Geometry check sheet. Reference: the model listing, model coordinates, mm. A direction names the side the tool comes from. Give positions to 0.01 mm unless a question says otherwise; leave off trailing zeros. Write each loop counter-clockwise with the first axis right and the second up, starting at its lowest first coordinate (ties: lowest second). Pieces come first, ordered by that corner, then holes.
(1) Cross-section at B-B (x = 8). Record the boundary of the cut face in (y, z), and give its area (3 significant figures).
(2) Tool access check on faces 5 (the flat face through (13, 27, -9)), 6 (the flat face through (30, -15, -2)). Record the directions out of +Z, -Z, +X, -X, +Y, -Y that give a thin tool (end or side, any length) a straight path to the whole face; none if there is none.
(3) Thickness scan on line 1 along Y through (x, z) = (8, -18.1); line 2 along X through (y, z) = (10, -38); line 3 along Y through (x, z) = (41, -2). Record the ranges inside material, lowest first.
(4) Depth check by flat-ended pin: P1, Ø3, axis at x = 33, z = -22.5, coming from the -Y side; P2, Ø2, axis at y = 10.5, z = -11, coming from the -X side; P3, Ø6, axis at y = 38.5, z = -32.5, coming from the +X side. Enter the tip coordinate at first touch or a pass-through.
(5) Cross-section at A-A (y = 10). Count the separate pieces of the cut face and the enclosed holes in it, and give its area (3 significant figures).
(6) Cross-section at C-C (y = 19). Record the boundary of the cut face in (x, z), and give its area (4 significant figures).
(7) Mould release check, pull along Y, two halves, no side actions. Record for faces 1 (the cylindrical face through (32.39, 24.43, -22.6)), 2 (the flat face through (12, 20, -20)), 3 (the flat face through (30, 55, -2)), 4 (the flat face through (33, 20, -22)): +Y half, -Y half, draft (parallel to the pull), parting line (faces both ways), or undercut.
(8) Cross-section at D-D (z = -43.5). Record the boundary of the cut face in (x, y).
```python
from build123d import *

# Parameters (mm, degrees)
SKETCH1_W                = 40
SKETCH1_H                = 40
BOSS_EXTRUDE1_DEPTH      = 40
SKETCH2_W                = 25
SKETCH2_H                = 20
CUT_EXTRUDE1_DEPTH       = 40
CHAMFER1_SIZE            = 15
CUT_EXTRUDE2_DEPTH       = 15
CHAMFER2_SIZE            = 4
SKETCH4_R                = 2.6
CUT_EXTRUDE3_DEPTH       = 17
BOSS_EXTRUDE2_DEPTH      = 8
BOSS_EXTRUDE2_DEPTH_BACK = 40
SKETCH5_W                = 40
SKETCH5_H                = 7
CHAMFER3_SIZE            = 35
CHAMFER3_SIZE2           = 25
CHAMFER4_SIZE            = 25
CHAMFER4_SIZE2           = 35
CHAMFER5_SIZE            = 8
FILLET1_R                = 10
FILLET2_R                = 5
SKETCH8_R                = 2.6
CUT_EXTRUDE4_DEPTH       = 34
BOSS_EXTRUDE3_DEPTH      = 20
FILLET3_R                = 4
FILLET4_R                = 2
CUT_EXTRUDE5_DEPTH       = 26
CHAMFER6_SIZE            = 2
CHAMFER6_SIZE2           = 10
FILLET5_R                = 2


with BuildPart() as part:
    # Sketch1 → Boss-Extrude1 (new body)
    with BuildSketch(Plane(origin=(0, 0, 0), x_dir=(1, 0, 0), z_dir=(0, 1, 0))):
        with Locations((20, 20)):
            Rectangle(SKETCH1_W, SKETCH1_H)
    extrude(amount=BOSS_EXTRUDE1_DEPTH)

    # Sketch2 → Cut-Extrude1 (cut)
    with BuildSketch(Plane(origin=(0, 40, 0), x_dir=(1, 0, 0), z_dir=(0, 1, 0))):
        with Locations((12.5, 30)):
            Rectangle(SKETCH2_W, SKETCH2_H)
    extrude(amount=-CUT_EXTRUDE1_DEPTH, mode=Mode.SUBTRACT)

    # Chamfer1
    chamfer1_edges = [part.edges().sort_by_distance(p)[0] for p in [
        (0, 20, 0),
    ]]
    chamfer(chamfer1_edges, length=CHAMFER1_SIZE)

    # Sketch3 → Cut-Extrude2 (cut)
    with BuildSketch(Plane.XY):
        Polygon((0, 10), (0, 15), (15, 15), (15, 5), (0, 5), align=None)
        Polygon((0, 30), (0, 25), (15, 25), (15, 35), (0, 35), align=None)
    extrude(amount=-CUT_EXTRUDE2_DEPTH, mode=Mode.SUBTRACT)

    # Chamfer2
    chamfer2_edges = [part.edges().sort_by_distance(p)[0] for p in [
        (15, 35, -7.5),
        (15, 25, -7.5),
        (15, 15, -7.5),
        (15, 5, -7.5),
    ]]
    chamfer(chamfer2_edges, length=CHAMFER2_SIZE)

    # Sketch4 → Cut-Extrude3 (cut)
    with BuildSketch(Plane.XY.offset(-15)):
        with Locations((8, 30)):
            Circle(SKETCH4_R)
        with Locations((8, 10)):
            Circle(SKETCH4_R)
    extrude(amount=-CUT_EXTRUDE3_DEPTH, mode=Mode.SUBTRACT)

    # Sketch5 → Boss-Extrude2 (add, two sides: drawn at the far end of the back side and taken through both)
    with BuildSketch(Plane(origin=(0, 0, -40), x_dir=(-1, 0, 0), z_dir=(0, 0, -1)).offset(-BOSS_EXTRUDE2_DEPTH_BACK)):
        with Locations((-60, 11.5)):
            Rectangle(SKETCH5_W, SKETCH5_H)
        with Locations((-60, 28.5)):
            Rectangle(SKETCH5_W, SKETCH5_H)
    extrude(amount=BOSS_EXTRUDE2_DEPTH + BOSS_EXTRUDE2_DEPTH_BACK)

    # Chamfer3
    chamfer3_edges = [part.edges().sort_by_distance(p)[0] for p in [
        (80, 28.5, 0),
    ]]
    chamfer3_side = [part.faces().sort_by_distance(p)[0] for p in [
        (39.166666667, 20, 0),
    ]]
    chamfer(chamfer3_edges, length=CHAMFER3_SIZE, length2=CHAMFER3_SIZE2, reference=chamfer3_side[0])

    # Chamfer4
    chamfer4_edges = [part.edges().sort_by_distance(p)[0] for p in [
        (80, 11.5, 0),
    ]]
    chamfer4_side = [part.faces().sort_by_distance(p)[0] for p in [
        (80, 11.5, -24),
    ]]
    chamfer(chamfer4_edges, length=CHAMFER4_SIZE, length2=CHAMFER4_SIZE2, reference=chamfer4_side[0])

    # Chamfer5
    chamfer5_edges = [part.edges().sort_by_distance(p)[0] for p in [
        (40, 28.5, -48),
        (40, 11.5, -48),
    ]]
    chamfer(chamfer5_edges, length=CHAMFER5_SIZE - 0.0001)  # a hair under: the kernel refuses the full size

    # Fillet1
    fillet1_edges = [part.edges().sort_by_distance(p)[0] for p in [
        (80, 11.5, -48),
        (80, 28.5, -48),
    ]]
    fillet(fillet1_edges, radius=FILLET1_R)

    # Fillet2
    fillet2_edges = [part.edges().sort_by_distance(p)[0] for p in [
        (80, 28.5, -25),
        (45, 28.5, 0),
        (45, 11.5, 0),
        (80, 11.5, -25),
        (47.9999, 28.5, -48),
        (47.9999, 11.5, -48),
    ]]
    fillet(fillet2_edges, radius=FILLET2_R)

    # Sketch8 → Cut-Extrude4 (cut)
    with BuildSketch(Plane(origin=(0, 32, 0), x_dir=(1, 0, 0), z_dir=(0, 1, 0))):
        with Locations(Location((70, 38, 0), (0, 0, 270))):
            Circle(SKETCH8_R)
    extrude(amount=-CUT_EXTRUDE4_DEPTH, mode=Mode.SUBTRACT)

    # Sketch9 → Boss-Extrude3 (add)
    with BuildSketch(Plane(origin=(40, 0, 0), x_dir=(0, 0, -1), z_dir=(1, 0, 0))):
        Polygon((0, 40), (0, 55), (4, 55), (20, 40), align=None)
        Polygon((0, 0), (0, -15), (4, -15), (20, 0), align=None)
    extrude(amount=-BOSS_EXTRUDE3_DEPTH)

    # Fillet3
    fillet3_edges = [part.edges().sort_by_distance(p)[0] for p in [
        (20, 55, -2),
        (40, 55, -2),
        (20, -15, -2),
        (40, -15, -2),
    ]]
    fillet(fillet3_edges, radius=FILLET3_R)

    # Fillet4
    fillet4_edges = [part.edges().sort_by_distance(p)[0] for p in [
        (32.5, 40, -40),
        (32.5, 0, -40),
    ]]
    fillet(fillet4_edges, radius=FILLET4_R)

    # Sketch10 → Cut-Extrude5 (cut)
    with BuildSketch(Plane(origin=(40, 0, 0), x_dir=(0, 0, -1), z_dir=(1, 0, 0))):
        Polygon((22, 15), (36, 15), (36, 20), (36, 25), (22, 25), align=None)
    extrude(amount=-CUT_EXTRUDE5_DEPTH, mode=Mode.SUBTRACT)

    # Chamfer6
    chamfer6_edges = [part.edges().sort_by_distance(p)[0] for p in [
        (40, 20, -36),
    ]]
    chamfer6_side = [part.faces().sort_by_distance(p)[0] for p in [
        (40, 20, -38),
    ]]
    chamfer(chamfer6_edges, length=CHAMFER6_SIZE, length2=CHAMFER6_SIZE2, reference=chamfer6_side[0])

    # Fillet5
    fillet5_edges = [part.edges().sort_by_distance(p)[0] for p in [
        (32.5, 25, -22),
        (27.5, 25, -36),
        (27.5, 15, -36),
        (32.5, 15, -22),
        (35, 25, -37),
        (35, 15, -37),
    ]]
    fillet(fillet5_edges, radius=FILLET5_R)


solid = part.part
```
Reply:
1. outline: (0, -20) - (7.4, -20) - (7.4, -15) - (5, -15) - (5, -7) - (0, -7) - close; (12.6, -20) - (27.4, -20) - (27.4, -15) - (25, -15) - (25, -7) - (15, -7) - (15, -15) - (12.6, -15) - close; (32.6, -20) - (40, -20) - (40, -7) - (35, -7) - (35, -15) - (32.6, -15) - close
1. area: 308 mm2
2. face 5: +Z, -X
2. face 6: +Z, -Z, +X, -X, -Y
3. line 1: y = 0 to 7.4, 12.6 to 27.4, 32.6 to 40
3. line 2: x = 25 to 67.4, 72.6 to 80
3. line 3: y = 8 to 15, 25 to 32
4. P1: stops at y = 0
4. P2: stops at x = 14.5
4. P3: stops at x = 40
5. separate pieces: 2
5. enclosed holes: 1
5. area: 2,260 mm2
6. outline: (0, -20) - (25, -20) - (25, -22) - (40, -22) - (40, 0) - (15, 0) - (0, -15) - close; (25, -40) - (40, -40) - (40, -38) - (30, -36) - (25, -36) - close
6. area: 767.5 mm2
7. face 1: undercut
7. face 2: draft
7. face 3: +Y half
7. face 4: undercut
8. outline: (43.5, 8) - (78.35, 8) - (78.35, 15) - (43.5, 15) - close; (43.5, 25) - (78.35, 25) - (78.35, 32) - (43.5, 32) - close
